```python
from build123d import *

# Parameters (mm, degrees)
SKETCH2_R           = 1.65
BOSS_EXTRUDE2_DEPTH = 3.175


with BuildPart() as part:
    # Sketch2 → Boss-Extrude2 (new body)
    with BuildSketch(Plane(origin=(0, 0, 0), x_dir=(1, 0, 0), z_dir=(0, 1, 0))):
        with BuildLine():
            Line((-38.1, -38.722993793), (-38.1, -58.722993793))
            ThreePointArc((-38.1, -58.722993793), (0, -70), (38.1, -58.722993793))
            Line((38.1, -58.722993793), (38.1, -38.722993793))
            Line((38.1, -38.722993793), (-38.1, -38.722993793))
        make_face()
        with Locations((-25.257106536, -60.976049146)):
            Circle(SKETCH2_R, mode=Mode.SUBTRACT)
        with Locations((25.257106536, -60.976049146)):
            Circle(SKETCH2_R, mode=Mode.SUBTRACT)
        with Locations((10.5, -58.722993793)):
            Circle(SKETCH2_R, mode=Mode.SUBTRACT)
        with Locations((-10.5, -58.722993793)):
            Circle(SKETCH2_R, mode=Mode.SUBTRACT)
    extrude(amount=BOSS_EXTRUDE2_DEPTH)


solid = part.part
```
Design review of the part built by this model. Coordinates are the model's own, in mm. Coordinates: 2 decimals unless noted, no trailing zeros. Loops run counter-clockwise (first coordinate to the right, second up) from the corner with the lowest first, then second, coordinate; pieces in that order, holes last. Notation, with made-up numbers: (21, -23) -> (26, -23) arc R29 ccw to (26, -3) -> close; hole circle Ø2 at (-37.5, -29.5). An arc over 180 degrees is marked (long way). Answer as a JSON object with one key per item and string values.
Q1. Take a section at D-D on x = 32. Give the boundary of the cut face in (y, z) (3 decimals), plus the area to 3 significant figures.
Answer block:
{"outline": "(0, 38.723) -> (3.175, 38.723) -> (3.175, 62.258) -> (0, 62.258) -> close", "area": "74.7 mm^2"}
Q2. Take a section at A-A on x = 10.5. Give the boundary of the cut face in (y, z) (3 decimals), plus the area to 3 significant figures.
Answer block:
{"outline": "(0, 38.723) -> (3.175, 38.723) -> (3.175, 57.073) -> (0, 57.073) -> close; (0, 60.373) -> (3.175, 60.373) -> (3.175, 69.208) -> (0, 69.208) -> close", "area": "86.3 mm^2"}
Q3. Take a section at C-C on x = -15.5. Give the boundary of the cut face in (y, z) (3 decimals), plus the area to 3 significant figures.
Answer block:
{"outline": "(0, 38.723) -> (3.175, 38.723) -> (3.175, 68.262) -> (0, 68.262) -> close", "area": "93.8 mm^2"}
Q4. Take a section at B-B on y = 1.1. Give the boundary of the cut face in (x, z).
Answer block:
{"outline": "(-38.1, 38.72) -> (38.1, 38.72) -> (38.1, 58.72) arc R70 ccw to (-38.1, 58.72) -> close; hole circle Ø3.3 at (-25.26, 60.98); hole circle Ø3.3 at (-10.5, 58.72); hole circle Ø3.3 at (10.5, 58.72); hole circle Ø3.3 at (25.26, 60.98)"}
Q5. The part is to be moulded in two halves that separate along Z. For faces 1 (the flat face through (1, 2, 38.723)), 2 (the flat face through (-1, 3.175, 54)), 3 (the cylindrical face through (-26.47, 1.57, 59.86)), say which applies: +Z half, -Z half, draft (parallel to the pull), parting line (faces both ways), or undercut.
Answer block:
{"face 1": "-Z half", "face 2": "draft", "face 3": "undercut"}
Q6. To check wall thickness, follow L1, parallel to X at y = 1.85, z = 60.5; L2, parallel to X at y = 2.45, z = 61; L3, parallel to Z at x = 11, y = 1.1. State the ranges of each line that lie inside material, in increasing order.
Answer block:
{"L1": "x = -35.21 to -26.84, -23.68 to 23.68, 26.84 to 35.21", "L2": "x = -34.34 to -26.91, -23.61 to 23.61, 26.91 to 34.34", "L3": "z = 38.72 to 57.15, 60.3 to 69.13"}
